Could you check a few things on this model? Use its own coordinates, in mm. Face numbers are marked on the shaded views. A direction names the side the tool comes from. Give positions to 0.01 mm unless a question says otherwise; leave off trailing zeros. Loops run counter-clockwise (first coordinate to the right, second up) from the corner with the lowest first, then second, coordinate; pieces in that order, holes last. Notation, with made-up numbers: (24, -2.75) -> (28, -2.75) arc R15 cw to (28, 12.25) -> close; hole circle Ø7 at (74.25, 87). An arc over 180 degrees is marked (long way). Write item = value, one per line. Start each with the question number.
1) I want a section at A-A (y = 9.5). List the corners of the cut face in (x, z) for me.
2) I need wall thicknesses on probe 1 along X at (y, z) = (10.3, 15); probe 2 along Y at (x, z) = (12.5, 9.75); probe 3 along X at (y, z) = (14, 7.5). Which ranges of each line are inside material? Lowest first, please. Write a range as from..to.
3) On a 3-axis mill with a long thin cutter (end or side, diameter ignored), from which of +Z, -Z, +X, -X, +Y, -Y can I reach the whole of each face in a straight line? I mean the marked faces 1, 2, 3 and 4. Say none if no direction works.
4) I'm going to push flat-ended pins straight in: pin 1 Ø4 at (x, z) = (22.5, 13.5) entering from -Y; pin 2 Ø5.5 at (x, z) = (22, 7) entering from +Y; pin 3 Ø1.5 at (x, z) = (-12, 10) entering from +Y. Where does each tip first touch, or does it pass through?
5) I want a section at B-B (x = 22.5). List the corners of the cut face in (y, z) for me.
6) I want a section at D-D (y = 3.5). List the corners of the cut face in (x, z) for me.
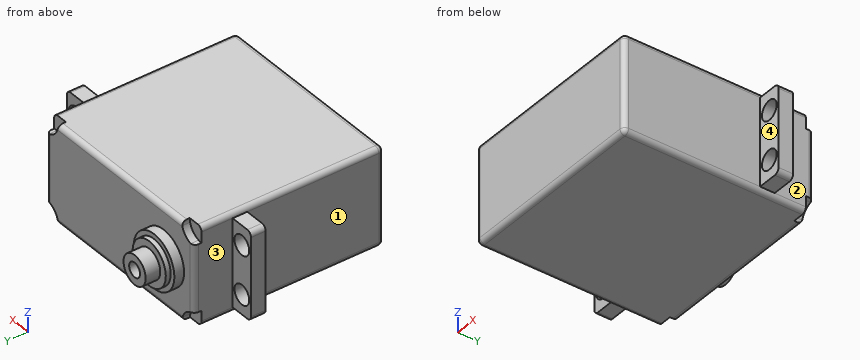
from build123d import *

# Parameters (mm, degrees)
SKETCH_1_W           = 40
SKETCH_1_H           = 39
EXTRUDE_1_DEPTH      = 20
SKETCH_2_R           = 3
EXTRUDE_2_DEPTH      = 6
SKETCH_2_5_R         = 5.5
SKETCH_2_5_R_2       = 4.5
EXTRUDE_5_DEPTH      = 2
SKETCH_2_6_R         = 4.5
SKETCH_2_6_R_2       = 3
EXTRUDE_6_DEPTH      = 3
SKETCH_2_8_W         = 0.8
SKETCH_2_8_H         = 0.8
CUT_EXTRUDE_5_DEPTH  = 1.61
SKETCH_2_12_W        = 0.8
SKETCH_2_12_H        = 0.8
CUT_EXTRUDE_6_DEPTH  = 1.61
FILLET_2_R           = 1
FILLET_3_R           = 1
FILLET_5_R           = 1
FILLET_6_R           = 1
FILLET_9_R           = 1
SKETCH_6_R           = 1.481108103
CUT_EXTRUDE_11_DEPTH = 3
SKETCH_7_W           = 18
SKETCH_7_H           = 3
EXTRUDE_10_DEPTH     = 5
SKETCH_14_R          = 2
CUT_EXTRUDE_12_DEPTH = 45.564559955
SKETCH_12_W          = 18
SKETCH_12_H          = 3
EXTRUDE_11_DEPTH     = 5
SKETCH_15_R          = 2
CUT_EXTRUDE_13_DEPTH = 45.564559955
FILLET_10_R          = 1


with BuildPart() as part:
    # Sketch 1 → Extrude 1 (new body)
    with BuildSketch(Plane.XY):
        Rectangle(SKETCH_1_W, SKETCH_1_H)
    extrude(amount=EXTRUDE_1_DEPTH)

    # Sketch 2 → Extrude 2 (add)
    with BuildSketch(Plane(origin=(0, 19.5, 0), x_dir=(1, 0, 0), z_dir=(0, 1, 0))):
        with Locations(Location((-11.898044795, -10, 0), (0, 0, 270))):
            Circle(SKETCH_2_R)
    extrude(amount=EXTRUDE_2_DEPTH)

    # Sketch 2_5 → Extrude 5 (add)
    with BuildSketch(Plane(origin=(0, 19.5, 0), x_dir=(1, 0, 0), z_dir=(0, 1, 0))):
        with Locations(Location((-11.898044795, -10, 0), (0, 0, 270))):
            Circle(SKETCH_2_5_R)
        with Locations(Location((-11.898044795, -10, 0), (0, 0, 270))):
            Circle(SKETCH_2_5_R_2, mode=Mode.SUBTRACT)
    extrude(amount=EXTRUDE_5_DEPTH)

    # Sketch 2_6 → Extrude 6 (add)
    with BuildSketch(Plane(origin=(0, 19.5, 0), x_dir=(1, 0, 0), z_dir=(0, 1, 0))):
        with Locations(Location((-11.898044795, -10, 0), (0, 0, 270))):
            Circle(SKETCH_2_6_R)
        with Locations(Location((-11.898044795, -10, 0), (0, 0, 270))):
            Circle(SKETCH_2_6_R_2, mode=Mode.SUBTRACT)
    extrude(amount=EXTRUDE_6_DEPTH)

    # Sketch 2_8 → Cut-Extrude 5 (cut)
    with BuildSketch(Plane(origin=(0, 19.5, 0), x_dir=(1, 0, 0), z_dir=(0, 1, 0))):
        with Locations((-19.6, -0.4)):
            Rectangle(SKETCH_2_8_W, SKETCH_2_8_H)
        with BuildLine():
            Line((-16.893747566, 0), (-19.2, 0))
            Line((-19.2, 0), (-19.2, -0.8))
            Line((-19.2, -0.8), (-16.998532995, -0.8))
            ThreePointArc((-16.998532995, -0.8), (-16.920055327, -0.403416654), (-16.893747566, 0))
        make_face()
        with BuildLine():
            Line((-16.998532995, -0.8), (-19.2, -0.8))
            Line((-19.2, -0.8), (-19.2, -3.001467005))
            ThreePointArc((-19.2, -3.001467005), (-17.80354784, -2.19645216), (-16.998532995, -0.8))
        make_face()
        with BuildLine():
            Line((-19.2, -3.001467005), (-19.2, -0.8))
            Line((-19.2, -0.8), (-20, -0.8))
            Line((-20, -0.8), (-20, -3.106252434))
            ThreePointArc((-20, -3.106252434), (-19.596583346, -3.079944673), (-19.2, -3.001467005))
        make_face()
    extrude(amount=-CUT_EXTRUDE_5_DEPTH, mode=Mode.SUBTRACT)

    # Sketch 2_12 → Cut-Extrude 6 (cut)
    with BuildSketch(Plane(origin=(0, 19.5, 0), x_dir=(1, 0, 0), z_dir=(0, 1, 0))):
        with Locations((19.6, -0.4)):
            Rectangle(SKETCH_2_12_W, SKETCH_2_12_H)
        with BuildLine():
            Line((20, -0.8), (19.2, -0.8))
            Line((19.2, -0.8), (19.2, -3.088057642))
            ThreePointArc((19.2, -3.088057642), (19.596765501, -3.164411784), (20, -3.19))
            Line((20, -3.19), (20, -0.8))
        make_face()
        with BuildLine():
            Line((19.2, -0.8), (16.911942358, -0.8))
            ThreePointArc((16.911942358, -0.8), (17.744329368, -2.255670632), (19.2, -3.088057642))
            Line((19.2, -3.088057642), (19.2, -0.8))
        make_face()
        with BuildLine():
            Line((19.2, 0), (16.81, 0))
            ThreePointArc((16.81, 0), (16.835588216, -0.403234499), (16.911942358, -0.8))
            Line((16.911942358, -0.8), (19.2, -0.8))
            Line((19.2, -0.8), (19.2, 0))
        make_face()
        with BuildLine():
            ThreePointArc((20, -16.81), (19.596765501, -16.835588216), (19.2, -16.911942358))
            Line((19.2, -16.911942358), (19.2, -19.2))
            Line((19.2, -19.2), (20, -19.2))
            Line((20, -19.2), (20, -16.81))
        make_face()
        with Locations((19.6, -19.6)):
            Rectangle(SKETCH_2_12_W, SKETCH_2_12_H)
        with BuildLine():
            Line((19.2, -19.2), (16.911942358, -19.2))
            ThreePointArc((16.911942358, -19.2), (16.835588216, -19.596765501), (16.81, -20))
            Line((16.81, -20), (19.2, -20))
            Line((19.2, -20), (19.2, -19.2))
        make_face()
        with BuildLine():
            ThreePointArc((19.2, -16.911942358), (17.744329368, -17.744329368), (16.911942358, -19.2))
            Line((16.911942358, -19.2), (19.2, -19.2))
            Line((19.2, -19.2), (19.2, -16.911942358))
        make_face()
        with BuildLine():
            Line((-16.911942358, -19.2), (-19.2, -19.2))
            Line((-19.2, -19.2), (-19.2, -20))
            Line((-19.2, -20), (-16.81, -20))
            ThreePointArc((-16.81, -20), (-16.835588216, -19.596765501), (-16.911942358, -19.2))
        make_face()
        with BuildLine():
            ThreePointArc((-16.911942358, -19.2), (-17.744329368, -17.744329368), (-19.2, -16.911942358))
            Line((-19.2, -16.911942358), (-19.2, -19.2))
            Line((-19.2, -19.2), (-16.911942358, -19.2))
        make_face()
        with BuildLine():
            Line((-19.2, -19.2), (-19.2, -16.911942358))
            ThreePointArc((-19.2, -16.911942358), (-19.596765501, -16.835588216), (-20, -16.81))
            Line((-20, -16.81), (-20, -19.2))
            Line((-20, -19.2), (-19.2, -19.2))
        make_face()
        with Locations((-19.6, -19.6)):
            Rectangle(SKETCH_2_12_W, SKETCH_2_12_H)
    extrude(amount=-CUT_EXTRUDE_6_DEPTH, mode=Mode.SUBTRACT)

    # Fillet 2
    fillet_2_edges = [part.edges().sort_by_distance(p)[0] for p in [
        (-0.041873783, 19.5, 0),
    ]]
    fillet(fillet_2_edges, radius=FILLET_2_R)

    # Fillet 3
    fillet_3_edges = [part.edges().sort_by_distance(p)[0] for p in [
        (-20, 19.5, 9.958126217),
        (0, 19.5, 20),
        (20, 19.5, 10),
    ]]
    fillet(fillet_3_edges, radius=FILLET_3_R)

    # Fillet 5
    fillet_5_edges = [part.edges().sort_by_distance(p)[0] for p in [
        (-20, -0.805, 0),
    ]]
    fillet(fillet_5_edges, radius=FILLET_5_R)

    # Fillet 6
    fillet_6_edges = [part.edges().sort_by_distance(p)[0] for p in [
        (20, -0.805, 0),
        (-20, -0.805, 20),
        (20, -0.805, 20),
    ]]
    fillet(fillet_6_edges, radius=FILLET_6_R)

    # Fillet 9
    fillet_9_edges = [part.edges().sort_by_distance(p)[0] for p in [
        (0, -19.5, 0),
        (-19.707106781, -19.5, 0.292893219),
        (-20, -19.5, 10),
        (20, -19.5, 10),
        (0, -19.5, 20),
        (-19.707106781, -19.5, 19.707106781),
        (19.707106781, -19.5, 19.707106781),
        (19.707106781, -19.5, 0.292893219),
    ]]
    fillet(fillet_9_edges, radius=FILLET_9_R)

    # Sketch 6 → Cut-Extrude 11 (cut)
    with BuildSketch(Plane(origin=(0, 25.5, 0), x_dir=(1, 0, 0), z_dir=(0, 1, 0))):
        with Locations(Location((-11.898044795, -10, 0), (0, 0, 270))):
            Circle(SKETCH_6_R)
    extrude(amount=-CUT_EXTRUDE_11_DEPTH, mode=Mode.SUBTRACT)

    # Sketch 7 → Extrude 10 (add)
    with BuildSketch(Plane(origin=(20, 0, 0), x_dir=(0, 0, -1), z_dir=(1, 0, 0))):
        with Locations((-10, 10)):
            Rectangle(SKETCH_7_W, SKETCH_7_H)
    extrude(amount=EXTRUDE_10_DEPTH)

    # Sketch 14 → Cut-Extrude 12 (cut, through all)
    with BuildSketch(Plane(origin=(0, 11.5, 0), x_dir=(1, 0, 0), z_dir=(0, 1, 0))):
        with Locations(Location((22.5, -5, 0), (0, 0, 270))):
            Circle(SKETCH_14_R)
        with Locations(Location((22.5, -15, 0), (0, 0, 270))):
            Circle(SKETCH_14_R)
    extrude(amount=-CUT_EXTRUDE_12_DEPTH, mode=Mode.SUBTRACT)

    # Sketch 12 → Extrude 11 (add)
    with BuildSketch(Plane.ZY.offset(20)):
        with Locations((10, 10)):
            Rectangle(SKETCH_12_W, SKETCH_12_H)
    extrude(amount=EXTRUDE_11_DEPTH)

    # Sketch 15 → Cut-Extrude 13 (cut, through all)
    with BuildSketch(Plane(origin=(0, 11.5, 0), x_dir=(1, 0, 0), z_dir=(0, 1, 0))):
        with Locations(Location((-22.5, -5, 0), (0, 0, 270))):
            Circle(SKETCH_15_R)
        with Locations(Location((-22.5, -15, 0), (0, 0, 270))):
            Circle(SKETCH_15_R)
    extrude(amount=-CUT_EXTRUDE_13_DEPTH, mode=Mode.SUBTRACT)

    # Fillet 10
    fillet_10_edges = [part.edges().sort_by_distance(p)[0] for p in [
        (25, 10, 19),
        (25, 10, 1),
        (-25, 10, 1),
        (-25, 10, 19),
    ]]
    fillet(fillet_10_edges, radius=FILLET_10_R)


solid = part.part
Answer list:
q1.outline = (-25, 2) arc R1 ccw to (-24, 1) -> (-20, 1) arc R1 ccw to (-19, 0) -> (19, 0) arc R1 ccw to (20, 1) -> (24, 1) arc R1 ccw to (25, 2) -> (25, 18) arc R1 ccw to (24, 19) -> (20, 19) arc R1 ccw to (19, 20) -> (-19, 20) arc R1 ccw to (-20, 19) -> (-24, 19) arc R1 ccw to (-25, 18) -> close; hole circle Ø4 at (-22.5, 5); hole circle Ø4 at (-22.5, 15); hole circle Ø4 at (22.5, 5); hole circle Ø4 at (22.5, 15)
q2.probe_1 = -25..-24.5, -20.5..20.5, 24.5..25
q2.probe_2 = -19.5..19.5
q2.probe_3 = -20..20
q3.face_1 = +Z, -Z, -X, -Y
q3.face_2 = +Z, -Z, +X, +Y
q3.face_3 = +Z, -Z, -X, +Y
q3.face_4 = +Z, -Z, +X, -Y
q4.pin_1 = 8.5
q4.pin_2 = 19.47
q4.pin_3 = 22.5
q5.outline = (8.5, 1) -> (11.5, 1) -> (11.5, 3) -> (8.5, 3) -> close; (8.5, 7) -> (11.5, 7) -> (11.5, 13) -> (8.5, 13) -> close; (8.5, 17) -> (11.5, 17) -> (11.5, 19) -> (8.5, 19) -> close
q6.outline = (-20, 1) arc R1 ccw to (-19, 0) -> (19, 0) arc R1 ccw to (20, 1) -> (20, 19) arc R1 ccw to (19, 20) -> (-19, 20) arc R1 ccw to (-20, 19) -> close
